Autodesk Fusion 360 part; units mm, degrees
sketch "Sketch15" plane through (0, 0, 0) normal (0, 1, 0) x (1, 0, 0)
  line L0 (0, 0) -> (-140, 0)
  line L1 (-140, 0) -> (-140, 120)
  line L2 (-140, 120) -> (0, 120)
  line L3 (0, 120) -> (0, 0)
  line L4 (0, 0) -> (-70, 0) construction
  line L5 (-70, 0) -> (-70, 102) construction
  line L6 (-70, 102) -> (-70, 153) construction
  line L7 (-70, 120) -> (-70, 0)
  arc A0 (-108.8844, 120) -> (-70, 102) centre (-70, 153) ccw
  arc A1 (-70, 102) -> (-140, 74.1889) centre (-70, 0) ccw
  dimension "d65" = 140
  dimension "d66" = 120
  dimension "d67" = 70
  dimension "d68" = 102
  dimension "d69" = 204
  dimension "d70" = 51
  dimension "d71" = 102
extrude "Extrude9" add sketch "Sketch15" along normal blind 70
ref_plane "WorkPlane3" through (-70, -34, -60) normal (0, 1, 0) x (0, 0, 1)
sketch "Sketch16" plane through (0, -34, 0) normal (0, 1, 0) x (1, 0, 0)
  line L0 (0, 0) -> (-70, 0) construction
  line L1 (-70, 0) -> (-70, 153) construction
  line L2 (-70, 0) -> (-70, 204)
  line L3 (-70, 0) -> (-172, 0)
  arc A0 (-70, 102) -> (-172, 0) centre (-70, 0) ccw
  arc A1 (-70, 204) -> (-70, 102) centre (-70, 153) ccw
  dimension "d75" = 70
  dimension "d76" = 153
  dimension "d77" = 204
  dimension "d78" = 102
revolve "Revolve6" cut sketch "Sketch16" angle 360 about axis through (-70, -34, 0) along (0, 0, -1)
fillet "Fillet1" radius 5 1 edges at (-70, 70, -120)
fillet "Fillet2" radius 5 3 edges at (-140, 32.5, -120) (-140, 68.5355, -118.5355) (-140, 70, -57.5)
fillet "Fillet3" radius 5 3 edges at (0, 32.5, -120) (0, 68.5355, -118.5355) (0, 70, -57.5)
Read the model definition and answer for the solid it produces. Units are mm, in the model's axes. Round coordinates to 2 decimals unless told otherwise and drop trailing zeros. Write each loop counter-clockwise with the first axis right and the second up, starting at its lowest first coordinate (ties: lowest second). Pieces come first, ordered by that corner, then holes. Notation, with made-up numbers: M 10,11 L 25,11 A23 ccw 25,37 Z; hole C 48,20.25 d8. An arc over 180 degrees is marked long. Use a Markdown table: item, result.
1) Straight lines are drawn through the part: line 1 along Z through (x, y) = (-27.5, 65.5); line 2 along X through (y, z) = (47, -35); line 3 along Z through (x, y) = (-53, 53). For each, find the intervals that lie inside material, in ascending order. Write a range as [from, to].
Answers follow:
| item | result |
|---|---|
| line 1 | z = [-119.97, 0] |
| line 2 | x = [-140, -121.17], [-18.83, 0] |
| line 3 | z = [-120, -50.46] |
2) A flat-ended cylindrical pin translates along its axis: pin 1 (1.5 mm diameter, centred on x = -101.5, y = 16.5, fed in from +Z). Find the tip coordinate at first contact, or state that the pin passes through.
Answers follow:
| item | result |
|---|---|
| pin 1 | stops at z = -82.29 |
3) The part is cut by section C-C (z = -72). Write down the section's boundary in (x, y).
Answers follow:
| item | result |
|---|---|
| outline | M -140,0 L -133.75,0 A72.25 cw -6.25,0 L 0,0 L 0,65 A5 ccw -5,70 L -135,70 A5 ccw -140,65 Z |
4) The part is cut by section A-A (y = 61). Write down the section's boundary in (x, z), plus the area to 3 significant figures.
Answers follow:
| item | result |
|---|---|
| outline | M -140,-115 A5 ccw -135,-120 L -5,-120 A5 ccw 0,-115 L 0,0 L -32.87,0 A37.13 cw -107.13,0 L -140,0 Z |
| area | 14,600 mm2 |
5) The part is cut by section B-B (x = -57.5). Write down the section's boundary in (y, z).
Answers follow:
| item | result |
|---|---|
| outline | M 0,-117.1 A49.44 cw 2.82,-120 L 65,-120 A5 ccw 70,-115 L 70,0 L 67.23,0 A101.23 cw 0,-95.35 Z |
6) The part is cut by section D-D (z = -31). Write down the section's boundary in (x, y), plus the area to 3 significant figures.
Answers follow:
| item | result |
|---|---|
| outline | M -140,33.4 A97.18 cw 0,33.4 L 0,65 A5 ccw -5,70 L -135,70 A5 ccw -140,65 Z |
| area | 2,240 mm2 |
